Check sheet for the modelled part. Datum: model origin and axes. Units: mm. A direction names the side the tool comes from. Coordinates: 2 decimals unless noted, no trailing zeros. Loops run counter-clockwise (first coordinate to the right, second up) from the corner with the lowest first, then second, coordinate; pieces in that order, holes last. Notation, with made-up numbers: M 6,20.5 L 35,20.5 A13 cw 35,24.5 Z; hole C 53.25,-14.75 d2. An arc over 180 degrees is marked long. Use CSV: the item, a comma, the result in double quotes. Start each with the question number.
(1) Section check C-C on x = -2. Record the cut outline in (y, z).
(2) Scan lines: line 1 (Y direction, x = 0, z = -1.5) (3 decimals); line 2 (X direction, y = 6, z = -3.05); line 3 (X direction, y = -2.5, z = -0.65) (3 decimals). Record each from-to range of solid material in increasing order.
(3) Section check D-D on y = 1. Record the cut outline in (x, z).
(4) Section check B-B on y = 5. Record the cut outline in (x, z), and give its area (4 significant figures).
(5) Go/stop test with flat-tipped pins: pin 1 Ø0.5 at (x, z) = (1, -2.5) entering from +Y; pin 2 Ø0.8 at (x, z) = (1, -3) entering from -Y; pin 3 Ø2 at (x, y) = (-4.5, -3.5) entering from -Z. Record where each tip stops, or that it passes through.
(6) Set-up check for faces 1 (the flat face through (-3.45, 0, -1)), 2 (the flat face through (3.45, 0, -1)), 3 (the cylindrical face through (-0.08, 10.75, -1.23)), 4 (the flat face through (1.625, -5, -2)), 5 (the flat face through (2.55, 5, -3)): record each of +Z, -Z, +X, -X, +Y, -Y from which the full face is reachable in a straight line by a thin tool's end or side.
(7) Draft check along X on faces 6 (the flat face through (0, 1.9, -3)), 7 (the cylindrical face through (0.08, -10.75, -1.23)), 8 (the flat face through (-4, 0, -2.5)). Enter one of: pulls with the +X half, pulls with the -X half, needs draft (parallel to the pull), parting line crosses it, or undercut.
(8) Section check A-A on z = -0.35. Record the cut outline in (x, y) (3 decimals).
from build123d import *

# Parameters (mm, degrees)
BOSS_EXTRUDE1_DEPTH = 2.5
SKETCH3_R           = 2.5
CUT_EXTRUDE1_DEPTH  = 4
SKETCH4_W           = 5.1
SKETCH4_H           = 6.2
BOSS_EXTRUDE2_DEPTH = 1
SKETCH5_W           = 5.1
SKETCH5_H           = 6.2
CUT_EXTRUDE2_DEPTH  = 0.55
CUT_EXTRUDE3_START  = -0.6
CUT_EXTRUDE3_DEPTH  = 0.6


with BuildPart() as part:
    # Sketch1 → Boss-Extrude1 (new body)
    with BuildSketch(Plane(origin=(0, 0, 0), x_dir=(0, 1, 0), z_dir=(0, 0, 1))):
        with BuildLine():
            Line((-7.3, 3.45), (7.3, 3.45))
            ThreePointArc((7.3, 3.45), (10.75, 0), (7.3, -3.45))
            Line((7.3, -3.45), (-7.3, -3.45))
            ThreePointArc((-7.3, -3.45), (-10.75, 0), (-7.3, 3.45))
        make_face()
    extrude(amount=-BOSS_EXTRUDE1_DEPTH)

    # Sketch3 → Cut-Extrude1 (cut)
    with BuildSketch(Plane.XY):
        with Locations((0, 5)):
            Circle(SKETCH3_R)
        with BuildLine():
            Line((-1.625, -7.5), (-1.625, -2))
            ThreePointArc((-1.625, -2), (0, -0.375), (1.625, -2))
            Line((1.625, -2), (1.625, -7.5))
            ThreePointArc((1.625, -7.5), (0, -9.125), (-1.625, -7.5))
        make_face()
    extrude(amount=-CUT_EXTRUDE1_DEPTH, mode=Mode.SUBTRACT)

    # Sketch4 → Boss-Extrude2 (add)
    with BuildSketch(Plane(origin=(0, 0, -2.5), x_dir=(1, 0, 0), z_dir=(0, 0, -1))):
        with BuildLine():
            Line((-5.45, 7.3), (-5.45, -7.3))
            ThreePointArc((-5.45, -7.3), (0, -12.75), (5.45, -7.3))
            Line((5.45, -7.3), (5.45, 7.3))
            ThreePointArc((5.45, 7.3), (0, 12.75), (-5.45, 7.3))
        make_face()
        with BuildLine():
            Line((1.625, 2), (1.625, 7.5))
            ThreePointArc((1.625, 7.5), (0, 9.125), (-1.625, 7.5))
            Line((-1.625, 7.5), (-1.625, 2))
            ThreePointArc((-1.625, 2), (0, 0.375), (1.625, 2))
        make_face(mode=Mode.SUBTRACT)
        with Locations((0, -5)):
            Rectangle(SKETCH4_W, SKETCH4_H, mode=Mode.SUBTRACT)
    extrude(amount=BOSS_EXTRUDE2_DEPTH)

    # Sketch5 → Cut-Extrude2 (cut)
    with BuildSketch(Plane(origin=(0, 0, -2.5), x_dir=(1, 0, 0), z_dir=(0, 0, -1))):
        with Locations((0, -5)):
            Rectangle(SKETCH5_W, SKETCH5_H)
    extrude(amount=-CUT_EXTRUDE2_DEPTH, mode=Mode.SUBTRACT)

    # Sketch6 → Cut-Extrude3 (cut)
    with BuildSketch(Plane(origin=(0, 0, -3.5), x_dir=(1, 0, 0), z_dir=(0, 0, -1)).offset(CUT_EXTRUDE3_START)):
        with BuildLine():
            Line((-5.45, -7.3), (-5.45, 7.3))
            ThreePointArc((-5.45, 7.3), (-4.924682731, 9.634523506), (-3.45, 11.519004622))
            Line((-3.45, 11.519004622), (-3.45, -11.519004622))
            ThreePointArc((-3.45, -11.519004622), (-4.924682731, -9.634523506), (-5.45, -7.3))
        make_face()
    extrude(amount=CUT_EXTRUDE3_DEPTH, mode=Mode.SUBTRACT)


solid = part.part
Outcome:
1,outline,"M -12.37,-3.5 L 1.9,-3.5 L 1.9,-1.95 L 3.5,-1.95 L 3.5,0 L -10.11,0 L -10.11,-2.5 L -12.37,-2.5 Z; M 6.5,-1.95 L 8.1,-1.95 L 8.1,-3.5 L 12.37,-3.5 L 12.37,-2.5 L 10.11,-2.5 L 10.11,0 L 6.5,0 Z"
2,line 1,"y = -10.75 to -9.125, -0.375 to 2.5, 7.5 to 10.75"
2,line 2,"x = -3.45 to -2.55, 2.55 to 5.45"
2,line 3,"x = -3.45 to -1.625, 1.625 to 3.45"
3,outline,"M -5.45,-2.9 L -3.45,-2.9 L -3.45,-3.5 L 5.45,-3.5 L 5.45,-2.5 L 3.45,-2.5 L 3.45,0 L -3.45,0 L -3.45,-2.5 L -5.45,-2.5 Z"
4,outline,"M -5.45,-2.9 L -3.45,-2.9 L -3.45,-3.5 L -2.55,-3.5 L -2.55,-1.95 L -2.5,-1.95 L -2.5,0 L -3.45,0 L -3.45,-2.5 L -5.45,-2.5 Z; M 2.5,-1.95 L 2.55,-1.95 L 2.55,-3.5 L 5.45,-3.5 L 5.45,-2.5 L 3.45,-2.5 L 3.45,0 L 2.5,0 Z"
4,area,"9.295 mm²"
5,pin 1,"stops at y = 12.7"
5,pin 2,"stops at y = -12.72"
5,pin 3,"stops at z = -2.9"
6,face 1,"+Z, -X, +Y, -Y"
6,face 2,"+Z, +X, +Y, -Y"
6,face 3,"+Z, +Y"
6,face 4,"+Z, -Z"
6,face 5,"-Z"
7,face 6,"undercut"
7,face 7,"parting line crosses it"
7,face 8,"needs draft"
8,outline,"M -3.45,-7.3 A3.45 ccw 3.45,-7.3 L 3.45,7.3 A3.45 ccw -3.45,7.3 Z; hole C 0,5 d5; hole M -1.625,-7.5 A1.625 ccw 1.625,-7.5 L 1.625,-2 A1.625 ccw -1.625,-2 Z"
